```python
from build123d import *

# Parameters (mm, degrees)
SKETCH2_W           = 61
SKETCH2_H           = 40.8
SKETCH2_R           = 1.6
BOSS_EXTRUDE1_DEPTH = 1.6
BOSS_EXTRUDE2_DEPTH = 25
SKETCH5_W           = 9.5
SKETCH5_H           = 12.3
BOSS_EXTRUDE3_DEPTH = 11.5
SKETCH6_R           = 3.5
BOSS_EXTRUDE4_DEPTH = 5
SKETCH7_R           = 3
BOSS_EXTRUDE5_DEPTH = 10
SKETCH8_W           = 10
SKETCH8_H           = 10
BOSS_EXTRUDE6_DEPTH = 14.5
CUT_EXTRUDE1_DEPTH  = 10


with BuildPart() as part:
    # Sketch2 → Boss-Extrude1 (new body)
    with BuildSketch(Plane.XY):
        Rectangle(SKETCH2_W, SKETCH2_H)
        with Locations((-27.4, 16.8)):
            Circle(SKETCH2_R, mode=Mode.SUBTRACT)
        with Locations((27.4, 16.8)):
            Circle(SKETCH2_R, mode=Mode.SUBTRACT)
        with Locations((-27.4, -17.4)):
            Circle(SKETCH2_R, mode=Mode.SUBTRACT)
        with Locations((27.4, -17.4)):
            Circle(SKETCH2_R, mode=Mode.SUBTRACT)
    extrude(amount=BOSS_EXTRUDE1_DEPTH)

    # Sketch3 → Boss-Extrude2 (add)
    with BuildSketch(Plane.XY.offset(1.6)):
        Polygon((-24, 19.4), (-24, 3.9), (-23.25, 3.9), (-23.25, 10.9), (-1.75, 10.9), (-1.75, 3.9), (-1, 3.9), (-1, 19.4), (-1.75, 19.4), (-1.75, 13.4), (-5.25, 13.4), (-5.25, 19.4), (-6, 19.4), (-6, 11.9), (-10, 11.9), (-10, 19.4), (-10.75, 19.4), (-10.75, 13.4), (-14.25, 13.4), (-14.25, 19.4), (-15, 19.4), (-15, 11.9), (-19, 11.9), (-19, 19.4), (-19.75, 19.4), (-19.75, 13.4), (-23.25, 13.4), (-23.25, 19.4), align=None)
        Polygon((14.25, 19.4), (14.25, 13.4), (10.75, 13.4), (10.75, 19.4), (10, 19.4), (10, 11.9), (6, 11.9), (6, 19.4), (5.25, 19.4), (5.25, 13.4), (1.75, 13.4), (1.75, 19.4), (1, 19.4), (1, 3.9), (1.75, 3.9), (1.75, 10.9), (23.25, 10.9), (23.25, 3.9), (24, 3.9), (24, 19.4), (23.25, 19.4), (23.25, 13.4), (19.75, 13.4), (19.75, 19.4), (19, 19.4), (19, 11.9), (15, 11.9), (15, 19.4), align=None)
    extrude(amount=BOSS_EXTRUDE2_DEPTH)

    # Sketch5 → Boss-Extrude3 (add)
    with BuildSketch(Plane.XY.offset(1.6)):
        with Locations((-7.25, -14.25)):
            Rectangle(SKETCH5_W, SKETCH5_H)
    extrude(amount=BOSS_EXTRUDE3_DEPTH)

    # Sketch6 → Boss-Extrude4 (add)
    with BuildSketch(Plane.XZ.offset(20.4)):
        with Locations(Location((-7.25, 8.45, 0), (0, 0, 90))):
            Circle(SKETCH6_R)
    extrude(amount=BOSS_EXTRUDE4_DEPTH)

    # Sketch7 → Boss-Extrude5 (add)
    with BuildSketch(Plane.XZ.offset(25.4)):
        with Locations(Location((-7.25, 8.45, 0), (0, 0, 270))):
            Circle(SKETCH7_R)
    extrude(amount=BOSS_EXTRUDE5_DEPTH)

    # Sketch8 → Boss-Extrude6 (add)
    with BuildSketch(Plane.XY.offset(1.6)):
        with Locations((-25.5, -1.4)):
            Rectangle(SKETCH8_W, SKETCH8_H)
        with Locations((25.5, -1.4)):
            Rectangle(SKETCH8_W, SKETCH8_H)
    extrude(amount=BOSS_EXTRUDE6_DEPTH)

    # Sketch9 → Cut-Extrude1 (cut)
    with BuildSketch(Plane.XZ.offset(6.4)):
        Polygon((-23.151020569, 16.1), (-20.5, 6.14534258), (-16.249696832, 6.089417538), (-15.914146582, 20.014752918), (-23.095095527, 19.846977793), align=None)
        Polygon((-29.415736124, 16.1), (-30.16614877, 9.208365841), (-30.5, 8.949622517), (-32.813418931, 7.814737758), (-35.128393598, 16.673480385), (-30.436281354, 21.104919727), align=None)
        Polygon((30.436281354, 21.104919727), (29.415736124, 16.1), (30.16614877, 9.208365841), (30.5, 8.949622517), (32.813418931, 7.814737758), (35.128393598, 16.673480385), align=None)
        Polygon((23.095095527, 19.846977793), (23.151020569, 16.1), (20.5, 6.14534258), (16.249696832, 6.089417538), (15.914146582, 20.014752918), align=None)
    extrude(amount=-CUT_EXTRUDE1_DEPTH, mode=Mode.SUBTRACT)


solid = part.part
```
Work out the finished part from the listing and answer in its coordinate system (mm). A direction names the side the tool comes from. Give positions to 0.01 mm unless a question says otherwise; leave off trailing zeros. Order: outer loops, then holes, each group sorted by start corner. A loop starts at its lowest first (then second) coordinate and runs counter-clockwise, first axis right, second up.
1. The mould has two halves that part along X. Classify faces 1 (the cylindrical face through (-4.72, -30.33, 6.84)), 2 (the flat face through (-1.75, 16, 14)), 3 (the flat face through (-5, -20.4, 3)), 4 (the flat face through (21.844, -1.47, 11.192)): released by +X, released by -X, zero draft, split by the parting line, or undercut.
Result sheet:
face 1: split by the parting line
face 2: undercut
face 3: zero draft
face 4: undercut
2. Straight lines are drawn through the part: L1, parallel to Y at x = 27.4, z = 1.3; L2, parallel to X at y = -13.5, z = 9.5; L3, parallel to Z at x = 15, y = 3. For each, find the intervals that lie inside material, in ascending order.
Result sheet:
L1: y = -20.4 to -19, -15.8 to 15.2, 18.4 to 20.4
L2: x = -12 to -2.5
L3: z = 0 to 1.6
3. For faces 5 (the flat face through (1, 12, 14)), 6 (the flat face through (24, 12, 14)), 7 (the flat face through (-21.844, -1.47, 11.192)), 8 (the flat face through (23.25, 16, 14)), determine the directions among +Z, -Z, +X, -X, +Y, -Y from which every point of the face is accessible in a straight line to the end or side of a thin tool.
Result sheet:
face 5: +Z, +Y, -Y
face 6: +Z, +X, +Y
face 7: +Z, -Y
face 8: +Z, +Y
4. Section B-B, the plane y = -17.4 is taken. Determine the outline of the cut face in (x, z), and give its area (3 significant figures).
Result sheet:
outline: (-30.5, 0) - (-29, 0) - (-29, 1.6) - (-30.5, 1.6) - close; (-25.8, 0) - (25.8, 0) - (25.8, 1.6) - (-2.5, 1.6) - (-2.5, 13.1) - (-12, 13.1) - (-12, 1.6) - (-25.8, 1.6) - close; (29, 0) - (30.5, 0) - (30.5, 1.6) - (29, 1.6) - close
area: 197 mm2
5. Each of these flat-tipped pins is pushed along its axis until it touches: P1, Ø3, axis at y = 15, z = 16, coming from the -X side; P2, Ø0.6, axis at x = 23.5, z = 8.5, coming from the +Y side; P3, Ø3, axis at x = -27, z = 12.5, coming from the +Y side. Where does it stop, or does it pass through?
Result sheet:
P1: stops at x = -24
P2: stops at y = 19.4
P3: stops at y = 3.6
6. Section C-C, the plane y = 9.5 is taken. Determine the outline of the cut face in (x, z), and give its area (3 significant figures).
Result sheet:
outline: (-30.5, 0) - (30.5, 0) - (30.5, 1.6) - (24, 1.6) - (24, 26.6) - (23.25, 26.6) - (23.25, 1.6) - (1.75, 1.6) - (1.75, 26.6) - (1, 26.6) - (1, 1.6) - (-1, 1.6) - (-1, 26.6) - (-1.75, 26.6) - (-1.75, 1.6) - (-23.25, 1.6) - (-23.25, 26.6) - (-24, 26.6) - (-24, 1.6) - (-30.5, 1.6) - close
area: 173 mm2
7. Section D-D, the plane z = 4 is taken. Give the number of separate pieces and of enclosed holes in the cut face, and give its area (3 significant figures).
Result sheet:
separate pieces: 5
enclosed holes: 0
area: 483 mm2
8. Section A-A, the plane x = -27.4 is taken. Determine the outline of the cut face in (y, z).
Result sheet:
outline: (-20.4, 0) - (-19, 0) - (-19, 1.6) - (-20.4, 1.6) - close; (-15.8, 0) - (15.2, 0) - (15.2, 1.6) - (3.6, 1.6) - (3.6, 16.1) - (-6.4, 16.1) - (-6.4, 1.6) - (-15.8, 1.6) - close; (18.4, 0) - (20.4, 0) - (20.4, 1.6) - (18.4, 1.6) - close
